Autodesk Inventor part; units mm, degrees
ref_plane "Arbeitsebene2" through (10, -17, 0) normal (1, 0, 0) x (0, 1, 0)
ref_plane "XZ Plane" through (0, 0, 0) normal (0, 1, 0) x (-1, 0, 0)
ref_plane "XY Plane" through (0, 0, 0) normal (0, 0, 1) x (1, 0, 0)
sketch "Sketch1" plane through (0, 0, 0) normal (0, 0, 1) x (1, 0, 0)
  line L0 (0, -35.8) -> (0, 40.5) construction
  line L1 (0, 0) -> (11.1575, 11.1575) construction
  line L2 (0, 0) -> (15.7791, 0) construction
  line L3 (0, 24.9) -> (14, 24.9)
  line L4 (14, 24.9) -> (14, 21.2415)
  line L5 (2.8009, -24.9) -> (14, -24.9)
  line L6 (14, -24.9) -> (14, -21.2415)
  line L7 (0, 24.9) -> (-14, 24.9)
  line L8 (-14, 24.9) -> (-14, 21.2415)
  line L9 (2.8009, -24.9) -> (-14, -24.9)
  line L10 (-14, -24.9) -> (-14, -21.2415)
  circle A0 centre (0, 0) radius 12.5
  line L11 (14, 24.9) -> (14, -21.2415)
  line L12 (-14, 21.2415) -> (-14, -21.2415)
  dimension "d0" = 45
  dimension "d5" = 25
  dimension "d19" = 28
extrude "Extrusion1" add sketch "Sketch1" along normal blind 5.5
sketch "Sketch2" plane through (0, 0, 5.5) normal (0, 0, 1) x (1, 0, 0)
  circle A0 centre (0, 0) radius 12.5
  line L0 (14, 24.9) -> (-14, 24.9)
  line L1 (-14, 24.9) -> (-14, -24.9)
  line L2 (-14, -24.9) -> (14, -24.9)
  line L3 (14, -24.9) -> (14, 24.9)
  line L4 (-37.0494, 0) -> (27.1749, 0) construction
  line L5 (0, -35.8) -> (0, 40.5) construction
  line L6 (-10, 21.9) -> (10, 21.9)
  line L7 (10, 21.9) -> (10, 18.9)
  line L8 (10, 18.9) -> (-10, 18.9)
  line L9 (-10, 18.9) -> (-10, 21.9)
  line L10 (-10, -21.9) -> (10, -21.9)
  line L11 (10, -21.9) -> (10, -18.9)
  line L12 (10, -18.9) -> (-10, -18.9)
  line L13 (-10, -18.9) -> (-10, -21.9)
  dimension "d8" = 20
  dimension "d9" = 3
  dimension "d10" = 3
  dimension "d20" = 18.9
  dimension "d21" = 18.9
extrude "Extrusion2" add sketch "Sketch2" along normal blind 7 contours L6 L7 L8 L9 | L13 L12 L11 L10
chamfer "Fase1" distance 0.7 distance2 7 1 edges at (0, 21.9, 12.5) measured on face at (-3.3333, 19.9, 12.5)
chamfer "Fase2" distance 0.7 distance2 7 1 edges at (0, -21.9, 12.5) measured on face at (-3.3333, -19.9, 12.5)
sketch "Skizze4" plane through (0, 0, 0) normal (0, 0, -1) x (-1, 0, 0)
  line L0 (10, -18.9) -> (-10, -18.9)
  line L1 (-10, 18.9) -> (10, 18.9)
  line L2 (10, -18.9) -> (-10, -18.9)
  line L3 (-10, -18.9) -> (-10, 18.9) construction
  line L4 (-10, 18.9) -> (10, 18.9)
  line L5 (10, 18.9) -> (10, -18.9)
  line L6 (-10, -21.9) -> (10, -21.9)
  line L7 (-10, -18.9) -> (10, -18.9)
  line L8 (10, -18.9) -> (10, -21.9)
  line L9 (10, -21.9) -> (-10, -21.9)
  line L10 (-10, -21.9) -> (-10, -18.9)
  point P0 (0, 0)
  point P1 (10, -20.4)
  point P2 (0, 0)
  point P3 (-10, -17)
  dimension "d22" = 18.9
  dimension "d23" = 20
  dimension "d24" = 3
  dimension "d33" = 17
ref_plane "Arbeitsebene2" through (10, -17, 0) normal (1, 0, 0) x (0, 1, 0)
sketch "Skizze5" plane through (10, -20.4, 0) normal (0, 0, -1) x (0, 1, 0)
  line L0 (50, 0.0005) -> (0, 0.0005)
  point P0 (20.4, -10)
  point P1 (25, 0)
  point P2 (40, 8)
  point P3 (6.6949, -37.8745)
  point P4 (0, 0.0005)
sketch "Skizze6" plane through (10, -17, 0) normal (1, 0, 0) x (0, 1, 0)
  line L0 (50, -0.1341) -> (0, -0.1341)
  line L1 (-5, 0.0159) -> (-5, 5.0159)
  line L2 (0, -0.1341) -> (0, 5.1659)
  line L3 (0, 1.0159) -> (2.1846, 1.0159)
  line L4 (-2.3, -1.5874) -> (-2.3, 1.1997)
  line L5 (0, -1.5874) -> (0, -0.1341)
  arc A0 (-2.3, 3.8322) -> (-0.8789, 0.0159) centre (0, 2.5159) ccw
  arc A1 (0, -0.1341) -> (0, 5.1659) centre (0, 2.5159) ccw
  line L6 (2.1846, 1.0159) -> (3.3346, -0.1341)
  line L7 (3.3346, -0.1341) -> (0, -0.1341)
  line L8 (0, 2.5159) -> (1.8859, 2.5159)
  line L9 (2.1846, 4.0159) -> (3.3346, 5.1659)
  line L10 (3.3346, 5.1659) -> (0, 5.1659)
  point P0 (17, 0)
  point P1 (25, 0)
  point P2 (40, 8)
  point P3 (6.6949, -37.8745)
  point P4 (0, -0.1341)
  dimension "d34" = 2.65
  dimension "d35" = 5
  dimension "d36" = 2.3
  dimension "d37" = 135
  dimension "d38" = 1.5
  dimension "d39" = 2.65
revolve "Umdrehung2" cut sketch "Skizze6" angle 360 about axis through (10, -17, -0.1341) along (0, 0, 1)
mirror "Spiegeln3" about plane through (0, 0, 0) normal (1, 0, 0) of "Umdrehung2"
mirror "Spiegeln4" about plane through (0, 0, 0) normal (0, 1, 0) of "Umdrehung2", "Spiegeln3"
properties part number "20_Cube_insert_Sample_holder"
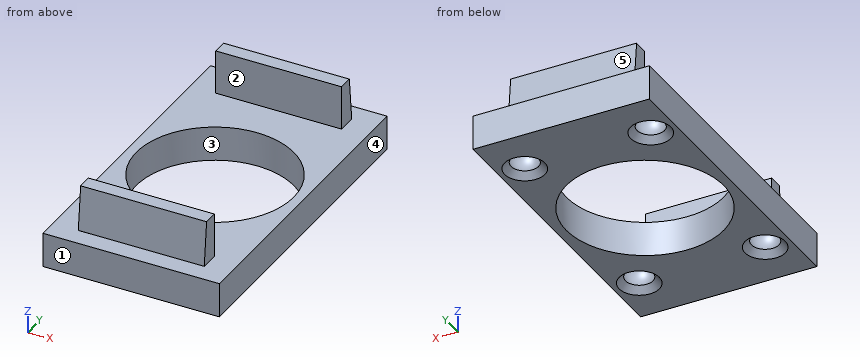
Geometry check sheet. Reference: the model listing, model coordinates, mm. Face numbers are marked on the shaded views. A direction names the side the tool comes from. Round coordinates to 2 decimals unless told otherwise and drop trailing zeros. Order: outer loops, then holes, each group sorted by start corner. A loop starts at its lowest first (then second) coordinate and runs counter-clockwise, first axis right, second up. Notation, with made-up numbers: M -35.75,60 L -18.75,60 A37 ccw -18.75,98 Z; hole C -4.5,33 d3. An arc over 180 degrees is marked long. Answer in a Markdown table with one row per item. Add a question column.
Item 1: Sectioned sample at A-A, the plane y = -0.5. Enter the section's corners in (x, z), plus the area to 3 significant figures.
Item 2: Sectioned sample at C-C, the plane z = 7. Enter the section's corners in (x, y).
Item 3: Depth check by flat-ended pin: pin 1 Ø7.5 at (x, y) = (11, 18.5) entering from -Z; pin 2 Ø2 at (x, y) = (-11.5, -16) entering from -Z; pin 3 Ø5.5 at (x, z) = (-2, 9.5) entering from -Y; pin 4 Ø3.5 at (y, z) = (-21, 7.5) entering from +X. Enter the tip coordinate at first touch or a pass-through.
Item 4: Draft check along X on the marked faces 3, 4 and 5. Enter one of: released by +X, released by -X, zero draft, split by the parting line, or undercut.
Item 5: Sectioned sample at D-D, the plane y = -17. Enter the section's corners in (x, z), plus the area to 3 significant figures.
Item 6: Set-up check for the marked faces 1 and 2: record each of +Z, -Z, +X, -X, +Y, -Y from which the full face is reachable in a straight line by a thin tool's end or side.
Item 7: Material ranges on L1, parallel to Y at x = 0, z = 2.95; L2, parallel to Y at x = -10.5, z = 1.5; L3, parallel to Z at x = -8.5, y = 18, recorded low to high. Write a range as [from, to].
Filled in:
| question | item | result |
|---|---|---|
| 1 | outline | M -14,0 L -12.49,0 L -12.49,5.5 L -14,5.5 Z; M 12.49,0 L 14,0 L 14,5.5 L 12.49,5.5 Z |
| 1 | area | 16.6 mm² |
| 2 | outline | M -10,-21.75 L 10,-21.75 L 10,-18.9 L -10,-18.9 Z; M -10,18.9 L 10,18.9 L 10,21.75 L -10,21.75 Z |
| 3 | pin 1 | stops at z = 0 |
| 3 | pin 2 | stops at z = 0.4 |
| 3 | pin 3 | stops at y = -21.78 |
| 3 | pin 4 | stops at x = 10 |
| 4 | face 3 | undercut |
| 4 | face 4 | released by +X |
| 4 | face 5 | zero draft |
| 5 | outline | M -14,0 L -13.2,0 L -12.18,1.02 A2.65 cw -12.18,4.02 L -13.33,5.17 L -6.67,5.17 L -7.82,4.02 A2.65 cw -7.82,1.02 L -6.8,0 L 6.8,0 L 7.82,1.02 A2.65 cw 7.82,4.02 L 6.67,5.17 L 13.33,5.17 L 12.18,4.02 A2.65 cw 12.18,1.02 L 13.2,0 L 14,0 L 14,5.5 L -14,5.5 Z |
| 5 | area | 100 mm² |
| 6 | face 1 | +Z, -Z, +X, -X, -Y |
| 6 | face 2 | +Z, +X, -X |
| 7 | L1 | y = [-24.9, -12.5], [12.5, 24.9] |
| 7 | L2 | y = [-24.9, -19.4], [-14.6, -6.78], [6.78, 14.6], [19.4, 24.9] |
| 7 | L3 | z = [5.17, 5.5] |
